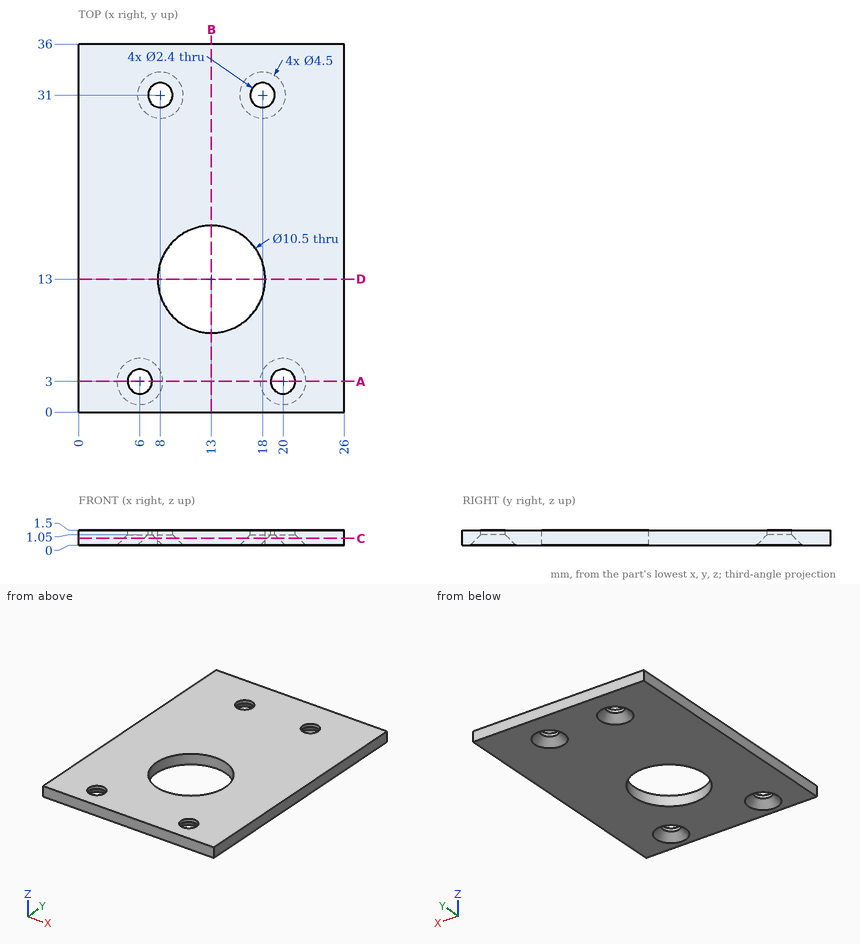
Source: three-view drawing plus pictorial views. Frame: mm from the lowest corner of the part. Coordinates: 2 decimals unless noted, no trailing zeros. Loops run counter-clockwise (first coordinate to the right, second up) from the corner with the lowest first, then second, coordinate; pieces in that order, holes last. Notation, with made-up numbers: (-16, -23.75) -> (5, -23.75) arc R22 ccw to (5, -17.75) -> close; hole circle Ø7 at (43.5, -38). An arc over 180 degrees is marked (long way). Answer in a Markdown table with one row per item. Add a question column.
Q1. Ray query, line 1 along X through (y, z) = (31, 1.2); line 2 along X through (y, z) = (3, 1.45); line 3 along Y through (x, z) = (13, 0.65). Return the intervals inside material, ascending.
Q2. Section A-A on y = 3. Return the cut outline in (x, z).
Q3. Section B-B on x = 13. Return the cut outline in (y, z), and give its area (4 significant figures).
Q4. Section D-D on y = 13. Return the cut outline in (x, z), and give its area (4 significant figures).
Q5. Section C-C on z = 0.7. Return the cut outline in (x, y).
Q6. Contact query for flat-ended pins moving along their axis: pin 1 Ø2 at (x, y) = (8, 31) entering from +Z; pin 2 Ø4 at (x, y) = (20, 3) entering from -Z. Output: stop coordinate, or through.
Computed values:
| question | item | result |
|---|---|---|
| 1 | line 1 | x = 0 to 6.8, 9.2 to 16.8, 19.2 to 26 |
| 1 | line 2 | x = 0 to 4.8, 7.2 to 18.8, 21.2 to 26 |
| 1 | line 3 | y = 0 to 7.75, 18.25 to 36 |
| 2 | outline | (0, 0) -> (3.75, 0) -> (4.8, 1.05) -> (4.8, 1.5) -> (0, 1.5) -> close; (7.2, 1.05) -> (8.25, 0) -> (17.75, 0) -> (18.8, 1.05) -> (18.8, 1.5) -> (7.2, 1.5) -> close; (21.2, 1.05) -> (22.25, 0) -> (26, 0) -> (26, 1.5) -> (21.2, 1.5) -> close |
| 3 | outline | (0, 0) -> (7.75, 0) -> (7.75, 1.5) -> (0, 1.5) -> close; (18.25, 0) -> (36, 0) -> (36, 1.5) -> (18.25, 1.5) -> close |
| 3 | area | 38.25 mm^2 |
| 4 | outline | (0, 0) -> (7.75, 0) -> (7.75, 1.5) -> (0, 1.5) -> close; (18.25, 0) -> (26, 0) -> (26, 1.5) -> (18.25, 1.5) -> close |
| 4 | area | 23.25 mm^2 |
| 5 | outline | (0, 0) -> (26, 0) -> (26, 36) -> (0, 36) -> close; hole circle Ø3.1 at (6, 3); hole circle Ø3.1 at (8, 31); hole circle Ø10.5 at (13, 13); hole circle Ø3.1 at (18, 31); hole circle Ø3.1 at (20, 3) |
| 6 | pin 1 | passes through |
| 6 | pin 2 | stops at z = 0.25 |
